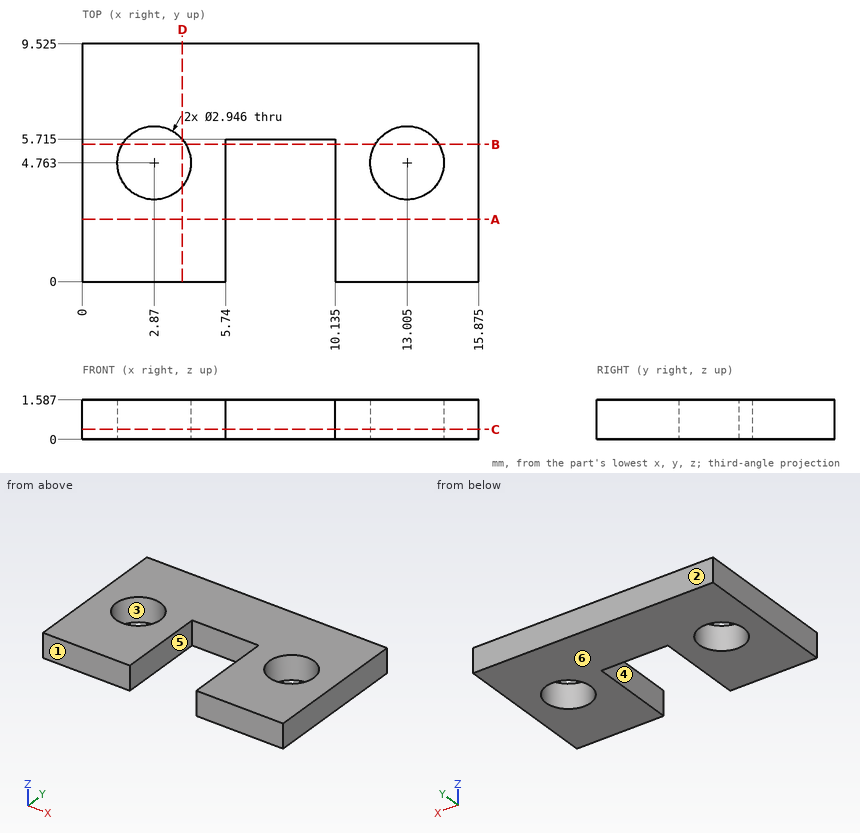
Verification items for this drawing (mm, ordinates from the low corner). A direction names the side the tool comes from. Coordinates: 2 decimals unless noted, no trailing zeros. Write each loop counter-clockwise with the first axis right and the second up, starting at its lowest first coordinate (ties: lowest second). Pieces come first, ordered by that corner, then holes. Notation, with made-up numbers: M -6.5,13 L 50.5,13 A9 ccw 50.5,26 Z; hole C -17.5,82.25 d9. An arc over 180 degrees is marked long. Answer as a JSON object with one key per item and string values.
1. Tool access check on the marked faces 5 and 6. Record the directions out of +Z, -Z, +X, -X, +Y, -Y that give a thin tool (end or side, any length) a straight path to the whole face; none if there is none.
Answers below:
{"face 5": "+Z, -Z, -Y", "face 6": "-Z, +X, -X, +Y, -Y"}
2. Section check A-A, the plane y = 2.5. Enter the section's corners in (x, z) (1 decimal).
Answers below:
{"outline": "M 0,0 L 5.7,0 L 5.7,1.6 L 0,1.6 Z; M 10.1,0 L 15.9,0 L 15.9,1.6 L 10.1,1.6 Z"}
3. Section check D-D, the plane x = 4. Enter the section's corners in (y, z) (1 decimal), plus the area to 3 significant figures.
Answers below:
{"outline": "M 0,0 L 3.8,0 L 3.8,1.6 L 0,1.6 Z; M 5.7,0 L 9.5,0 L 9.5,1.6 L 5.7,1.6 Z", "area": "12.1 mm²"}
4. Section check B-B, the plane y = 5.5. Enter the section's corners in (x, z) (1 decimal).
Answers below:
{"outline": "M 0,0 L 1.6,0 L 1.6,1.6 L 0,1.6 Z; M 4.1,0 L 5.7,0 L 5.7,1.6 L 4.1,1.6 Z; M 10.1,0 L 11.7,0 L 11.7,1.6 L 10.1,1.6 Z; M 14.3,0 L 15.9,0 L 15.9,1.6 L 14.3,1.6 Z"}
5. Scan lines: L1, parallel to X at y = 5.5, z = 1.35 (1 decimal); L2, parallel to X at y = 3.25, z = 0.1 (1 decimal); L3, parallel to X at y = 3.75, z = 1.15 (1 decimal). Record each from-to range of solid material in increasing order.
Answers below:
{"L1": "x = 0 to 1.6, 4.1 to 5.7, 10.1 to 11.7, 14.3 to 15.9", "L2": "x = 0 to 5.7, 10.1 to 15.9", "L3": "x = 0 to 1.8, 3.9 to 5.7, 10.1 to 11.9, 14.1 to 15.9"}
6. Draft check along Y on the marked faces 1, 2, 3 and 4. Enter one of: released by +Y, released by -Y, zero draft, split by the parting line, or undercut.
Answers below:
{"face 1": "released by -Y", "face 2": "released by +Y", "face 3": "undercut", "face 4": "zero draft"}
7. Section check C-C, the plane z = 0.4. Enter the section's corners in (x, y) (1 decimal).
Answers below:
{"outline": "M 0,0 L 5.7,0 L 5.7,5.7 L 10.1,5.7 L 10.1,0 L 15.9,0 L 15.9,9.5 L 0,9.5 Z; hole C 2.9,4.8 d2.9; hole C 13,4.8 d2.9"}
